from build123d import *

# Parameters (mm, degrees)
SKETCH9_W           = 36
SKETCH9_H           = 36
BOSS_EXTRUDE1_DEPTH = 40
CHAMFER2_SIZE       = 18
SKETCH10_W          = 36
SKETCH10_H          = 40
BOSS_EXTRUDE2_DEPTH = 8
SKETCH12_W          = 44
SKETCH12_H          = 40
BOSS_EXTRUDE3_DEPTH = 8
CHAMFER3_SIZE       = 18
CHAMFER4_SIZE       = 6
SKETCH13_W          = 36.769552622
SKETCH13_H          = 20
CUT_EXTRUDE6_DEPTH  = 39.59798
SKETCH14_R          = 3
CUT_EXTRUDE7_DEPTH  = 70.512588881
SKETCH15_R          = 7.1
CUT_EXTRUDE8_DEPTH  = 5.2
CUT_EXTRUDE9_START  = -5.2
SKETCH16_R          = 7.1
CUT_EXTRUDE9_DEPTH  = 5.2
BOSS_EXTRUDE4_DEPTH = 20
FILLET1_R           = 2
SKETCH19_R          = 2.25
CUT_EXTRUDE10_DEPTH = 70.512588881
SKETCH20_R          = 2.8
CUT_EXTRUDE11_DEPTH = 7
SKETCH21_R          = 4
CUT_EXTRUDE12_DEPTH = 4
SKETCH22_R          = 2.1
CUT_EXTRUDE13_DEPTH = 6
SKETCH23_W          = 11.455844123
SKETCH23_H          = 40
CUT_EXTRUDE14_DEPTH = 6
CHAMFER5_SIZE       = 3


with BuildPart() as part:
    # Sketch9 → Boss-Extrude1 (new body)
    with BuildSketch(Plane(origin=(0, 0, 0), x_dir=(1, 0, 0), z_dir=(0, 1, 0))):
        with Locations((18, 18)):
            Rectangle(SKETCH9_W, SKETCH9_H)
    extrude(amount=BOSS_EXTRUDE1_DEPTH)

    # Chamfer2
    chamfer2_edges = [part.edges().sort_by_distance(p)[0] for p in [
        (0, 20, -36),
    ]]
    chamfer(chamfer2_edges, length=CHAMFER2_SIZE)

    # Sketch10 → Boss-Extrude2 (add)
    with BuildSketch(Plane(origin=(36, 0, 0), x_dir=(0, 0, -1), z_dir=(1, 0, 0))):
        with Locations((18, 20)):
            Rectangle(SKETCH10_W, SKETCH10_H)
    extrude(amount=BOSS_EXTRUDE2_DEPTH)

    # Sketch12 → Boss-Extrude3 (add)
    with BuildSketch(Plane.XY):
        with Locations((22, 20)):
            Rectangle(SKETCH12_W, SKETCH12_H)
    extrude(amount=BOSS_EXTRUDE3_DEPTH)

    # Chamfer3
    chamfer3_edges = [part.edges().sort_by_distance(p)[0] for p in [
        (44, 20, -36),
        (0, 20, 8),
    ]]
    chamfer(chamfer3_edges, length=CHAMFER3_SIZE)

    # Chamfer4
    chamfer4_edges = [part.edges().sort_by_distance(p)[0] for p in [
        (44, 20, 8),
    ]]
    chamfer(chamfer4_edges, length=CHAMFER4_SIZE)

    # Sketch13 → Cut-Extrude6 (cut)
    with BuildSketch(Plane(origin=(23, 0, 23), x_dir=(0.7071067811865465, 0, -0.7071067811865487), z_dir=(0.7071067811865487, 0, 0.7071067811865465))):
        with Locations((25.455844123, 22)):
            Rectangle(SKETCH13_W, SKETCH13_H)
    extrude(amount=-CUT_EXTRUDE6_DEPTH, mode=Mode.SUBTRACT)

    # Sketch14 → Cut-Extrude7 (cut, through all)
    with BuildSketch(Plane(origin=(0, 40, 0), x_dir=(1, 0, 0), z_dir=(0, 1, 0))):
        with Locations(Location((32, 4, 0), (0, 0, 270))):
            Circle(SKETCH14_R)
    extrude(amount=-CUT_EXTRUDE7_DEPTH, mode=Mode.SUBTRACT)

    # Sketch15 → Cut-Extrude8 (cut)
    with BuildSketch(Plane(origin=(0, 12, 0), x_dir=(1, 0, 0), z_dir=(0, 1, 0))):
        with Locations(Location((32, 4, 0), (0, 0, 270))):
            Circle(SKETCH15_R)
    extrude(amount=-CUT_EXTRUDE8_DEPTH, mode=Mode.SUBTRACT)

    # Sketch16 → Cut-Extrude9 (cut)
    with BuildSketch(Plane(origin=(0, 32, 0), x_dir=(-1, 0, 0), z_dir=(0, -1, 0)).offset(CUT_EXTRUDE9_START)):
        with Locations(Location((-32, 4, 0), (0, 0, 270))):
            Circle(SKETCH16_R)
    extrude(amount=CUT_EXTRUDE9_DEPTH, mode=Mode.SUBTRACT)

    # Sketch18 → Boss-Extrude4 (add)
    with BuildSketch(Plane(origin=(0, 12, 0), x_dir=(1, 0, 0), z_dir=(0, 1, 0))):
        Polygon((40.464466094, 21.535533906), (34.807611845, 15.878679656), (44, 6.686291501), (44, 18), align=None)
        Polygon((14.464466094, -4.464466094), (20.121320344, 1.192388155), (29.313708499, -8), (18, -8), align=None)
    extrude(amount=BOSS_EXTRUDE4_DEPTH)

    # Fillet1
    fillet1_edges = [part.edges().sort_by_distance(p)[0] for p in [
        (14.464466094, 22, 4.464466094),
        (29.313708499, 22, 8),
        (20.121320344, 22, -1.192388155),
        (44, 22, -6.686291501),
        (40.464466094, 22, -21.535533906),
        (34.807611845, 22, -15.878679656),
    ]]
    fillet(fillet1_edges, radius=FILLET1_R)

    # Sketch19 → Cut-Extrude10 (cut, through all)
    with BuildSketch(Plane(origin=(0, 40, 0), x_dir=(1, 0, 0), z_dir=(0, 1, 0))):
        with Locations(Location((12, 8, 0), (0, 0, 270))):
            Circle(SKETCH19_R)
        with Locations(Location((28, 24, 0), (0, 0, 270))):
            Circle(SKETCH19_R)
    extrude(amount=-CUT_EXTRUDE10_DEPTH, mode=Mode.SUBTRACT)

    # Sketch20 → Cut-Extrude11 (cut)
    with BuildSketch(Plane(origin=(0, 0, 0), x_dir=(-1, 0, 0), z_dir=(0, -1, 0))):
        with Locations(Location((-12, 8, 0), (0, 0, 90))):
            Circle(SKETCH20_R)
        with Locations(Location((-28, 24, 0), (0, 0, 90))):
            Circle(SKETCH20_R)
    extrude(amount=-CUT_EXTRUDE11_DEPTH, mode=Mode.SUBTRACT)

    # Sketch21 → Cut-Extrude12 (cut)
    with BuildSketch(Plane(origin=(0, 40, 0), x_dir=(1, 0, 0), z_dir=(0, 1, 0))):
        with Locations(Location((28, 24, 0), (0, 0, 270))):
            Circle(SKETCH21_R)
        with Locations(Location((12, 8, 0), (0, 0, 270))):
            Circle(SKETCH21_R)
    extrude(amount=-CUT_EXTRUDE12_DEPTH, mode=Mode.SUBTRACT)

    # Sketch22 → Cut-Extrude13 (cut)
    with BuildSketch(Plane(origin=(-9, 0, -9), x_dir=(-0.7071067811865487, 0, 0.7071067811865465), z_dir=(-0.7071067811865465, 0, -0.7071067811865487))):
        with Locations((-15.455844123, 36)):
            Circle(SKETCH22_R)
        with Locations((-35.455844123, 36)):
            Circle(SKETCH22_R)
        with Locations((-35.455844123, 4)):
            Circle(SKETCH22_R)
        with Locations((-15.455844123, 4)):
            Circle(SKETCH22_R)
    extrude(amount=-CUT_EXTRUDE13_DEPTH, mode=Mode.SUBTRACT)

    # Sketch23 → Cut-Extrude14 (cut)
    with BuildSketch(Plane(origin=(-9, 0, -9), x_dir=(-0.7071067811865487, 0, 0.7071067811865465), z_dir=(-0.7071067811865465, 0, -0.7071067811865487))):
        with Locations((-25.455844123, 20)):
            Rectangle(SKETCH23_W, SKETCH23_H)
    extrude(amount=-CUT_EXTRUDE14_DEPTH, mode=Mode.SUBTRACT)

    # Chamfer5
    chamfer5_edges = [part.edges().sort_by_distance(p)[0] for p in [
        (17.292893219, 6, -26.807611845),
        (9.192388155, 6, -18.707106781),
    ]]
    chamfer(chamfer5_edges, length=CHAMFER5_SIZE)


solid = part.part
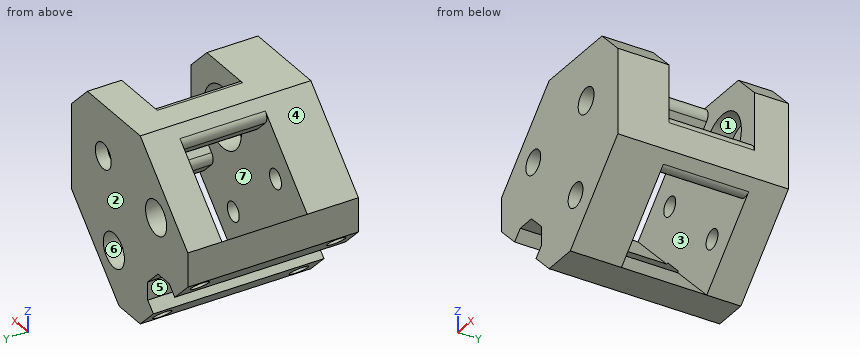
For this review, take the finished solid that the model builds, in its own axes (mm). Face numbers are marked on the shaded views. A direction names the side the tool comes from. Give positions to 0.01 mm unless a question says otherwise; leave off trailing zeros. Loops run counter-clockwise (first coordinate to the right, second up) from the corner with the lowest first, then second, coordinate; pieces in that order, holes last. Notation, with made-up numbers: M 69.5,24.25 L 106.5,24.25 A6 ccw 106.5,35.25 Z; hole C 68.25,0 d11. An arc over 180 degrees is marked long. Put each result on its own line as item: value. Start each with the question number.
(1) Machinability: for the marked faces 5, 6 and 7, which of the approach directions +Z, -Z, +X, -X, +Y, -Y give a long, thin tool a straight path to every point of the face, cutting with its end or side? Answer none if there is none.
(2) Wall thickness on L1, parallel to Y at x = 23.5, z = 1.5; L2, parallel to Y at x = 35, z = -3.5; L3, parallel to Z at x = 29.5, y = 33: over which ranges is each line inside the solid? List them lowest first.
(3) Add section B-B, the plane x = 28. Give the number of separate pieces and of enclosed holes in the cut face, then the cut area to 3 significant figures.
(4) Add section A-A, the plane y = 22.5. Write out the cut boundary in (x, z), then the cut area to 3 significant figures.
(5) Add section C-C, the plane y = 33. Write out the cut boundary in (x, z).
(6) The part is to be moulded in two halves that separate along Y. For the marked faces 1, 2, 3 and 4, say which applies: +Y half, -Y half, draft (parallel to the pull), parting line (faces both ways), or undercut.
(7) For pin 1 (3.5 mm diameter, centred on y = 11.5, z = -27, fed in from -X); pin 2 (1.3 mm diameter, centred on x = 9.5, y = 24.5, fed in from -Z); pin 3 (6 mm diameter, centred on y = 8.5, z = -23.5, fed in from -X); pin 4 (2.5 mm diameter, centred on x = 12, z = -8, fed in from -Y), all flat-tipped, find the tip position at first contact; note any pin that passes through.
Result:
1. face 5: -X, +Y, -Y
1. face 6: +Y
1. face 7: none
2. L1: y = 0 to 12, 32 to 40
2. L2: y = 0 to 6.8, 37.2 to 40
2. L3: z = -32.5 to -25.68, -22.32 to -10.65, 2.65 to 8
3. separate pieces: 4
3. enclosed holes: 0
3. area: 606 mm^2
4. outline: M 0,-18 L 4.95,-22.95 L 7.07,-20.83 L 10.83,-20.83 L 0,-10 Z; M 13.05,-31.05 L 18,-36 L 26,-36 L 15.17,-25.17 L 15.17,-28.93 Z; M 15.88,3.05 L 18.71,0.22 A2 ccw 21.54,0.22 L 25.9,4.59 A2 ccw 24.49,8 L 18,8 L 15.88,5.88 A2 ccw Z; M 36.22,-17.29 L 39.05,-20.12 A2 ccw 41.88,-20.12 L 44,-18 L 44,-11.51 A2 ccw 40.59,-10.1 L 36.22,-14.46 A2 ccw Z
4. area: 249 mm^2
5. outline: M 0,-18 L 4.95,-22.95 L 7.07,-20.83 L 11.31,-20.83 L 15.17,-24.69 L 15.17,-28.93 L 13.05,-31.05 L 18,-36 L 26,-36 L 44,-18 L 44,2 L 38,8 L 18,8 L 0,-10 Z; hole C 12,-8 d4.5; hole C 32,-4 d14.2; hole C 28,-24 d4.5
6. face 1: undercut
6. face 2: +Y half
6. face 3: undercut
6. face 4: draft
7. pin 1: stops at x = 15.17
7. pin 2: stops at z = -20.83
7. pin 3: stops at x = 2.5
7. pin 4: passes through
